Autodesk Inventor part; units mm, degrees
ref_plane "YZ Plane" through (0, 0, 0) normal (1, 0, 0) x (0, 1, 0)
ref_plane "XZ Plane" through (0, 0, 0) normal (0, 1, 0) x (-1, 0, 0)
ref_plane "XY Plane" through (0, 0, 0) normal (0, 0, 1) x (1, 0, 0)
sketch "스케치1" plane through (0, 0, 0) normal (0, 1, 0) x (-1, 0, 0)
  line L0 (0, 0) -> (11, 0)
  line L1 (11, 0) -> (11, -4)
  line L2 (11, -4) -> (0, -4)
  line L3 (0, -4) -> (0, 0)
  dimension "d0" = 11
  dimension "d1" = 4
extrude "돌출1" add sketch "스케치1" along normal blind 7
sketch "스케치2" plane through (0, 7, 0) normal (0, 1, 0) x (1, 0, 0)
  line L0 (0, 0) -> (0, 4) construction
  line L1 (0, 2) -> (-11, 2) construction
  line L2 (-11, 4) -> (-11, 0) construction
  point P0 (-1.3, 2)
  point P1 (-4.3, 2)
  point P2 (-7.5, 2)
  point P3 (-9.7, 2)
  point P4 (-4.3, 2)
  dimension "d59" = 1.3
  dimension "d60" = 2.2
  dimension "d61" = 3.2
  dimension "d62" = 1.3
  dimension "d69" = 0
hole "구멍1" at (-9.7, 7, -2) direction (0, -1, 0) diameter 0.65 end through all
hole "구멍2" at (-7.5, 7, -2) direction (0, -1, 0) diameter 1.3 end through all
hole "구멍3" at (-4.3, 7, -2) direction (0, -1, 0) diameter 0.67 end through all
hole "구멍4" at (-1.3, 7, -2) direction (0, -1, 0) diameter 1 depth 5.8 tip angle 90 countersink diameter 1.3 countersink angle 3
sketch "스케치3" plane through (0, 7, 0) normal (0, 1, 0) x (1, 0, 0)
  circle A0 centre (-4.3, 2) radius 1
  circle A1 centre (-4.3, 2) radius 0.335
  point P0 (0, 0)
  point P1 (-4.3, 2)
  dimension "d50" = 2
extrude "돌출2" add sketch "스케치3" along normal blind 1.5
sketch "스케치4" plane through (0, 0, 0) normal (0, -1, 0) x (1, 0, 0)
  circle A0 centre (-4.3, -2) radius 1
  circle A1 centre (-4.3, -2) radius 0.335
  point P0 (0, 0)
  point P1 (-4.3, -2)
  dimension "d53" = 2
extrude "돌출3" add sketch "스케치4" along normal blind 1.5
sketch "스케치5" plane through (0, 0, -4) normal (0, 0, -1) x (-1, 0, 0)
  point P0 (0, 0)
equation "\"d8\" = G23_F"
equation "\"d15\" = Screw_F"
equation "\"d22\" = G23_M"
equation "\"G23_F\" = 0.65"
equation "\"G23_M\" = 0.67"
equation "\"Screw_F\" = 1.3"
equation "\"Screw_M\" = 1.6"
properties part number "BOt"
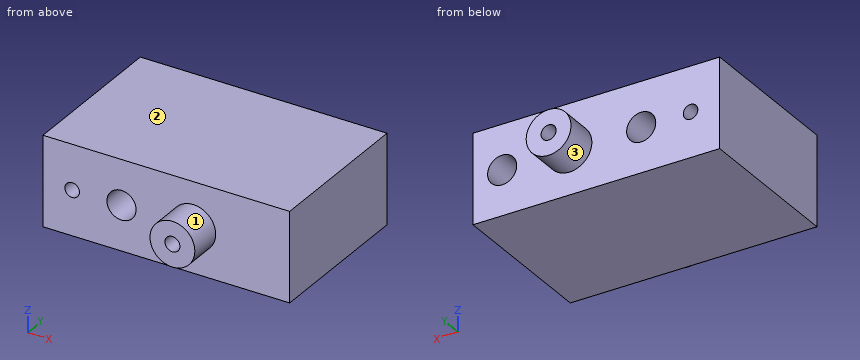
CAD build for the part. Positions are in the model's coordinates, mm. Face numbers are marked on the shaded views. A direction names the side the tool comes from. Round coordinates to 2 decimals unless told otherwise and drop trailing zeros. Order: outer loops, then holes, each group sorted by start corner. A loop starts at its lowest first (then second) coordinate and runs counter-clockwise, first axis right, second up.
Q1. Slice it at A-A (x = -4.3). Write the cut outline in (y, z) (3 decimals), and give its area (3 significant figures).
Q2. Slice it at B-B (y = 1). Write the cut outline in (x, z) (3 decimals), and give its area (3 significant figures).
Q3. Which spindle directions (+Z, -Z, +X, -X, +Y, -Y) get a long thin tool onto all of the face, cutting with end or side? Do the marked faces 1, 2 and 3. Say none if no direction does.
Q4. Wall check: L1, parallel to Z at x = -1, y = 4.5; L2, parallel to Z at x = -4.3, y = 1.25 (3 decimals); L3, parallel to X at y = 3.75, z = -2 (3 decimals). Give the ranges that are in metal, low to high.
Q5. Slice it at D-D (y = -0.5). Write the cut outline in (x, z) (3 decimals), and give its area (3 significant figures).
Q6. Drop flat-ended pins along their axis: pin 1 (1 mm diameter, centred on x = -6, z = -1.5, fed in from +Y); pin 2 (2 mm diameter, centred on x = -6.5, z = -1.5, fed in from -Y). Give the stop position or say it passes through.
Q7. Slice it at C-C (z = -1.2). Write the cut outline in (x, y), and give its area (3 significant figures).
Results below:
1. outline: (-1.5, -3) - (0, -3) - (0, -4) - (7, -4) - (7, -3) - (8.5, -3) - (8.5, -2.335) - (-1.5, -2.335) - close; (-1.5, -1.665) - (8.5, -1.665) - (8.5, -1) - (7, -1) - (7, 0) - (0, 0) - (0, -1) - (-1.5, -1) - close
1. area: 27.3 mm2
2. outline: (-11, -4) - (0, -4) - (0, 0) - (-11, 0) - close; hole circle Ø0.65 at (-9.7, -2); hole circle Ø1.3 at (-7.5, -2); hole circle Ø0.67 at (-4.3, -2); hole circle Ø0.6 at (-1.3, -2)
2. area: 41.7 mm2
3. face 1: -Y
3. face 2: +Z, +X, -X, +Y, -Y
3. face 3: +Y
4. L1: z = -4 to -2.5, -1.5 to 0
4. L2: z = -4 to -2.335, -1.665 to 0
4. L3: x = -11 to -10.025, -9.375 to -8.15, -6.85 to -4.635, -3.965 to -1.865, -0.735 to 0
5. outline: circle Ø2 at (-4.3, -2); hole circle Ø0.67 at (-4.3, -2)
5. area: 2.79 mm2
6. pin 1: stops at y = 7
6. pin 2: stops at y = 0
7. outline: (-11, 0) - (-4.9, 0) - (-4.9, -1.5) - (-3.7, -1.5) - (-3.7, 0) - (0, 0) - (0, 7) - (-3.7, 7) - (-3.7, 8.5) - (-4.9, 8.5) - (-4.9, 7) - (-11, 7) - close
7. area: 80.6 mm2
